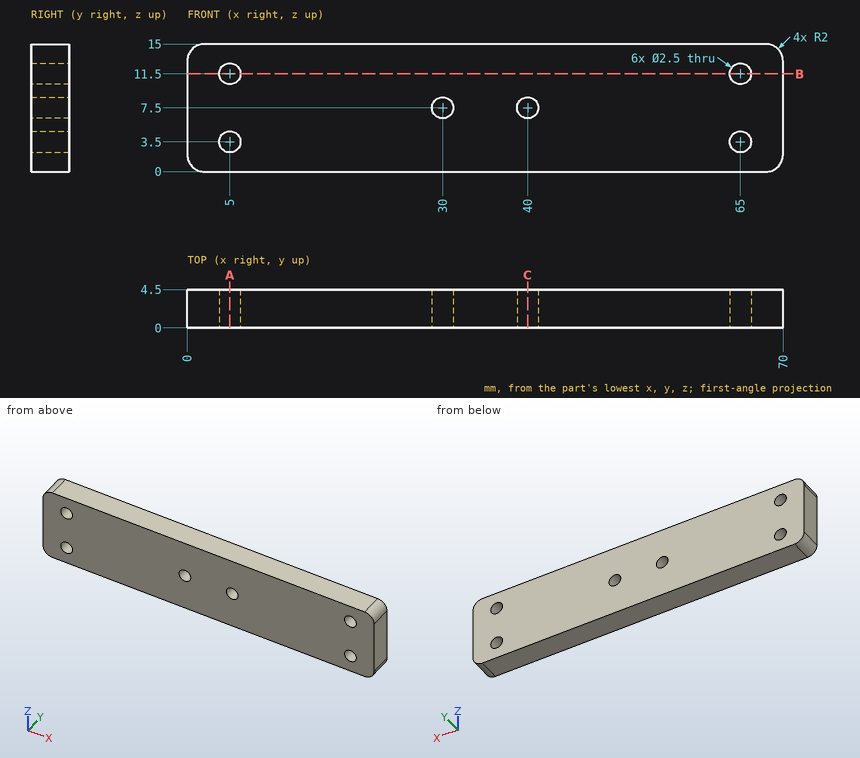
Geometry: see drawing. Coordinates: mm, zero at the bounding-box minimum. Give positions to 0.01 mm unless a question says otherwise; leave off trailing zeros. Loops run counter-clockwise (first coordinate to the right, second up) from the corner with the lowest first, then second, coordinate; pieces in that order, holes last. Notation, with made-up numbers: (-34.75, -9) - (-7.75, -9) arc R10 ccw to (-7.75, 5) - close; hole circle Ø3 at (-28, -35). An arc over 180 degrees is marked (long way). Answer as CSV lines item,"result". Start each with the question number.
1. Section C-C, the plane x = 40. Return loops of the section in (y, z), plus the area to 4 significant figures.
2. Ray query, L1, parallel to X at y = 0.9, z = 11.5; L2, parallel to Z at x = 65, y = 2.7; L3, parallel to X at y = 2, z = 7.5. Return the intervals inside material, ascending.
3. Pin query (flat end, axial travel): P1, Ø2, axis at x = 65, z = 11.5, coming from the -Y side; P2, Ø4, axis at x = 40, z = 7.5, coming from the -Y side. Return the tip coordinate at first contact, or that it passes through.
4. Section A-A, the plane x = 5. Return loops of the section in (y, z).
5. Section B-B, the plane z = 11.5. Return loops of the section in (x, y).
Answers:
1,outline,"(0, 0) - (4.5, 0) - (4.5, 6.25) - (0, 6.25) - close; (0, 8.75) - (4.5, 8.75) - (4.5, 15) - (0, 15) - close"
1,area,"56.25 mm2"
2,L1,"x = 0 to 3.75, 6.25 to 63.75, 66.25 to 70"
2,L2,"z = 0 to 2.25, 4.75 to 10.25, 12.75 to 15"
2,L3,"x = 0 to 28.75, 31.25 to 38.75, 41.25 to 70"
3,P1,"passes through"
3,P2,"stops at y = 0"
4,outline,"(0, 0) - (4.5, 0) - (4.5, 2.25) - (0, 2.25) - close; (0, 4.75) - (4.5, 4.75) - (4.5, 10.25) - (0, 10.25) - close; (0, 12.75) - (4.5, 12.75) - (4.5, 15) - (0, 15) - close"
5,outline,"(0, 0) - (3.75, 0) - (3.75, 4.5) - (0, 4.5) - close; (6.25, 0) - (63.75, 0) - (63.75, 4.5) - (6.25, 4.5) - close; (66.25, 0) - (70, 0) - (70, 4.5) - (66.25, 4.5) - close"
